Read the model definition and answer for the solid it produces. Units are mm, in the model's axes. A direction names the side the tool comes from. Coordinates: 2 decimals unless noted, no trailing zeros. Write each loop counter-clockwise with the first axis right and the second up, starting at its lowest first coordinate (ties: lowest second). Pieces come first, ordered by that corner, then holes.
(1) The part is cut by section B-B, the plane y = -3. Determine the outline of the cut face in (x, z), and give its area (3 significant figures).
(2) Straight lines are drawn through the part: line 1 along X through (y, z) = (2, 19); line 2 along Z through (x, y) = (63, 1.8); line 3 along Z through (x, y) = (39, -30). For each, find the intervals that lie inside material, in ascending order.
(3) Determine the mould class of faces 1 (the flat face through (88.2, -44, 2)), 2 (the flat face through (47, 4.5, 24)), 3 (the flat face through (77.8, -44, 2)), 4 (the flat face through (0, -11.7, 3.7)) for opening direction X: pulls with the +X half, pulls with the -X half, needs draft (parallel to the pull), parting line crosses it, or undercut.
(4) The part is cut by section C-C, the plane y = -42. Determine the outline of the cut face in (x, z), and give its area (3 significant figures).
(5) Which of the six approach directions +Z, -Z, +X, -X, +Y, -Y give full straight-line access (tool end or side, diameter ignored) to faces 5 (the flat face through (49, -34, 4)), 6 (the flat face through (7.8, -44, 2)), 7 (the conical face through (45.639, -20.925, 1.094))?
(6) The part is cut by section A-A, the plane x = 33. Determine the outline of the cut face in (y, z).
(7) The part is cut by section D-D, the plane x = 16. State how many separate pieces and enclosed holes the cut face has, and give its area (3 significant figures).
(8) Given pin 1 (10 mm diameter, centred on x = 78, z = 19, fed in from -Y); pin 2 (8.5 mm diameter, centred on x = 18, y = -23.5, fed in from +Z); pin 3 (6 mm diameter, centred on x = 46, y = -15, fed in from +Z), each flat-ended and moving along its own axis, determine where each tip first touches the part or whether it passes through.
```python
from build123d import *

# Parameters (mm, degrees)
SKETCH_1_W                  = 96
SKETCH_1_H                  = 47
EXTRUDE_1_DEPTH             = 4
SKETCH_12_W                 = 96
SKETCH_12_H                 = 4
SKETCH_12_R                 = 4.4
EXTRUDE_3_DEPTH             = 4.5
SKETCH_12_4_R               = 4.4
CUT_EXTRUDE_1_DEPTH         = 0.5
SKETCH_2_R                  = 5.2
CUT_EXTRUDE_2_DEPTH         = 10
HOLE_WIZARD_M6_1_AT_2_COUNT = 2
HOLE_WIZARD_M6_1_AT_2_PITCH = 30
HOLE_WIZARD_M6_1_AT_3_COUNT = 2
HOLE_WIZARD_M6_1_AT_3_PITCH = 60
FILLET_1_R                  = 0.5


with BuildPart() as part:
    # Sketch 1 → Extrude 1 (new body)
    with BuildSketch(Plane.XY):
        with Locations((48, -23.5)):
            Rectangle(SKETCH_1_W, SKETCH_1_H)
    extrude(amount=EXTRUDE_1_DEPTH)

    # Sketch 12 → Extrude 3 (add)
    # profile 1 of 2: a face of its own
    with BuildSketch(Plane(origin=(0, 0, 0), x_dir=(1, 0, 0), z_dir=(0, 1, 0))):
        with Locations((48, -2)):
            Rectangle(SKETCH_12_W, SKETCH_12_H)
    # profile 2 of 2: a face of its own
    with BuildSketch(Plane(origin=(0, 0, 0), x_dir=(1, 0, 0), z_dir=(0, 1, 0))):
        Polygon((96, -4), (0, -4), (0, -5), (0, -39), (96, -39), align=None)
        with Locations(Location((18, -19, 0), (0, 0, 270))):
            Circle(SKETCH_12_R, mode=Mode.SUBTRACT)
        with Locations(Location((33, -19, 0), (0, 0, 270))):
            Circle(SKETCH_12_R, mode=Mode.SUBTRACT)
        with Locations(Location((48, -19, 0), (0, 0, 270))):
            Circle(SKETCH_12_R, mode=Mode.SUBTRACT)
        with BuildLine():
            ThreePointArc((67.4, -19), (63, -23.4), (58.6, -19))
            ThreePointArc((58.6, -19), (63, -14.6), (67.4, -19))
        make_face(mode=Mode.SUBTRACT)
        with BuildLine():
            ThreePointArc((82.4, -19), (78, -23.4), (73.6, -19))
            ThreePointArc((73.6, -19), (78, -14.6), (82.4, -19))
        make_face(mode=Mode.SUBTRACT)
    extrude(amount=EXTRUDE_3_DEPTH)

    # Sketch 12_4 → Cut-Extrude 1 (cut)
    with BuildSketch(Plane(origin=(0, 0, 0), x_dir=(1, 0, 0), z_dir=(0, 1, 0))):
        Polygon((96, -4), (0, -4), (0, -5), (0, -39), (96, -39), align=None)
        with Locations(Location((18, -19, 0), (0, 0, 270))):
            Circle(SKETCH_12_4_R, mode=Mode.SUBTRACT)
        with Locations(Location((33, -19, 0), (0, 0, 270))):
            Circle(SKETCH_12_4_R, mode=Mode.SUBTRACT)
        with Locations(Location((48, -19, 0), (0, 0, 270))):
            Circle(SKETCH_12_4_R, mode=Mode.SUBTRACT)
        with BuildLine():
            ThreePointArc((67.4, -19), (63, -23.4), (58.6, -19))
            ThreePointArc((58.6, -19), (63, -14.6), (67.4, -19))
        make_face(mode=Mode.SUBTRACT)
        with BuildLine():
            ThreePointArc((82.4, -19), (78, -23.4), (73.6, -19))
            ThreePointArc((73.6, -19), (78, -14.6), (82.4, -19))
        make_face(mode=Mode.SUBTRACT)
    extrude(amount=CUT_EXTRUDE_1_DEPTH, mode=Mode.SUBTRACT)

    # Sketch 2 → Cut-Extrude 2 (cut)
    with BuildSketch(Plane.XY.offset(4)):
        with Locations((13, -6)):
            Circle(SKETCH_2_R)
        with Locations((13, -41)):
            Circle(SKETCH_2_R)
        with Locations((83, -41)):
            Circle(SKETCH_2_R)
        with Locations((83, -6)):
            Circle(SKETCH_2_R)
        with BuildLine():
            Line((77.8, -41), (77.8, -47))
            Line((77.8, -47), (88.2, -47))
            Line((88.2, -47), (88.2, -41))
            ThreePointArc((88.2, -41), (83, -46.2), (77.8, -41))
        make_face()
        with BuildLine():
            Line((7.8, -47), (18.2, -47))
            Line((18.2, -47), (18.2, -41))
            ThreePointArc((18.2, -41), (13, -46.2), (7.8, -41))
            Line((7.8, -41), (7.8, -47))
        make_face()
    extrude(amount=-CUT_EXTRUDE_2_DEPTH, mode=Mode.SUBTRACT)

    # Sketch 15 → Hole Wizard M6 _1 (revolve, cut)
    with BuildSketch(Plane(origin=(18, -23.5, 4), x_dir=(0, -1, 0), z_dir=(1, 0, 0))):
        Polygon((0, 0), (0, 4), (3.3, 4), (3.3, 3.1), (6.4, 0), align=None)
    hole_wizard_m6_1 = revolve(axis=Axis((18, -23.5, 10.35), (0, 0, -1)), mode=Mode.SUBTRACT)

    # Hole Wizard M6 _1 at 2: Hole Wizard M6 _1 ×2
    with Locations(*[(i * HOLE_WIZARD_M6_1_AT_2_PITCH, 0, 0) for i in range(1, HOLE_WIZARD_M6_1_AT_2_COUNT)]):
        add(hole_wizard_m6_1, mode=Mode.SUBTRACT)

    # Hole Wizard M6 _1 at 3: Hole Wizard M6 _1 ×2
    with Locations(*[(i * HOLE_WIZARD_M6_1_AT_3_PITCH, 0, 0) for i in range(1, HOLE_WIZARD_M6_1_AT_3_COUNT)]):
        add(hole_wizard_m6_1, mode=Mode.SUBTRACT)

    # Fillet 1
    fillet_1_edges = [part.edges().sort_by_distance(p)[0] for p in [
        (96, 2.5, 39),
        (0, 2.5, 39),
        (96, -47, 2),
        (0, -47, 2),
    ]]
    fillet(fillet_1_edges, radius=FILLET_1_R)


solid = part.part
```
Computed:
1. outline: (0, 0) - (8.75, 0) - (8.75, 4) - (0, 4) - close; (17.25, 0) - (78.75, 0) - (78.75, 4) - (17.25, 4) - close; (87.25, 0) - (96, 0) - (96, 4) - (87.25, 4) - close
1. area: 316 mm2
2. line 1: x = 0 to 13.6, 22.4 to 28.6, 37.4 to 43.6, 52.4 to 58.6, 67.4 to 73.6, 82.4 to 96
2. line 2: z = 0 to 14.6, 23.4 to 39
2. line 3: z = 0 to 4
3. face 1: undercut
3. face 2: needs draft
3. face 3: undercut
3. face 4: pulls with the -X half
4. outline: (0, 0) - (7.8, 0) - (7.8, 4) - (0, 4) - close; (18.2, 0) - (77.8, 0) - (77.8, 4) - (18.2, 4) - close; (88.2, 0) - (96, 0) - (96, 4) - (88.2, 4) - close
4. area: 301 mm2
5. face 5: +Z, +X, -X, -Y
5. face 6: +Z, -Z, -Y
5. face 7: +Z
6. outline: (-47, 0) - (4.5, 0) - (4.5, 14.6) - (0.5, 14.6) - (0.5, 4) - (-47, 4) - close; (0.5, 23.4) - (4.5, 23.4) - (4.5, 39) - (0.5, 39) - close
7. separate pieces: 4
7. enclosed holes: 0
7. area: 208 mm2
8. pin 1: stops at y = 0.5
8. pin 2: stops at z = 1.85
8. pin 3: stops at z = 4
